Input: part model. Units: mm. Frame: model coordinates. Face numbers are marked on the shaded views. Coordinates: 2 decimals unless noted, no trailing zeros. Order: outer loops, then holes, each group sorted by start corner. A loop starts at its lowest first (then second) coordinate and runs counter-clockwise, first axis right, second up. Notation, with made-up numbers: M 58,-16 L 81,-16 A29 cw 81,9 Z; hole C -21,-34.5 d1. An arc over 180 degrees is marked long. Answer in a Markdown table with one row per item.
Autodesk Inventor part; units mm, degrees
ref_plane "YZ Plane" through (0, 0, 0) normal (1, 0, 0) x (0, 1, 0)
ref_plane "XZ Plane" through (0, 0, 0) normal (0, 1, 0) x (-1, 0, 0)
ref_plane "XY Plane" through (0, 0, 0) normal (0, 0, 1) x (1, 0, 0)
sketch "Sketch2" plane through (0, 0, 0) normal (1, 0, 0) x (0, 1, 0)
  circle A0 centre (0, 0) radius 10
  circle A1 centre (0, 0) radius 12.5
  dimension "d3" = 20
  dimension "d4" = 25
extrude "Extrusion1" add sketch "Sketch2" along normal blind 25
sketch "Sketch3" plane through (0, 0, 0) normal (-1, 0, 0) x (0, 0, 1)
  circle A0 centre (0, 0) radius 10
  arc A1 (10, 0) -> (-10, 0) centre (0, 0) ccw
  circle A2 centre (0, 0) radius 12.5
  arc A3 (12.5, 0) -> (-12.5, 0) centre (0, 0) ccw
  line L0 (-12.5, 0) -> (-10, 0)
  line L1 (10, 0) -> (12.5, 0)
revolve "Revolution1" add sketch "Sketch3" angle 180 about axis through (0, 0, 10) along (0, 0, 1) picked at (-11.4487, 1.7949) contours A0 L0 A2 L1
sketch "Sketch5" plane through (25, 0, 0) normal (1, 0, 0) x (0, 0, -1)
  circle A0 centre (-8, 8) radius 1
  point P0 (0, 0)
  dimension "d9" = 2
extrude "Extrusion2" add sketch "Sketch5" along normal blind 7
mirror "Mirror1" about plane through (0, 0, 0) normal (0, 0, 1) of "Extrusion2"
mirror "Mirror2" about plane through (0, 0, 0) normal (0, 1, 0) of "Extrusion2", "Mirror1"
properties part number "Plasmid Half 1"
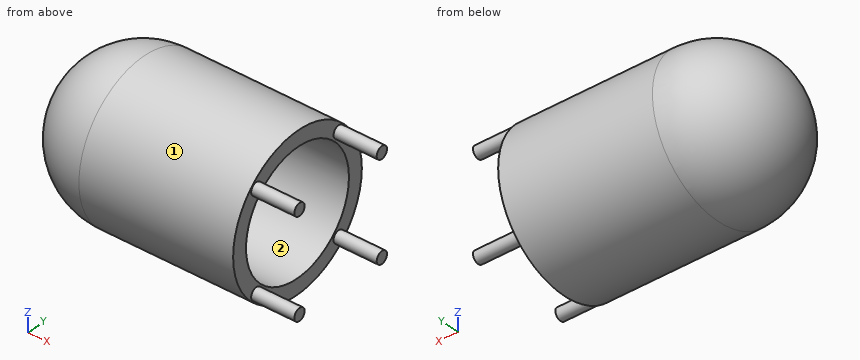
1) Contact query for flat-ended pins moving along their axis: pin 1 (4 mm diameter, centred on x = 4, y = 7, fed in from +Z); pin 2 (8 mm diameter, centred on y = -5, z = -2, fed in from -X); pin 3 (4 mm diameter, centred on x = 10, y = 9.5, fed in from -Z). Output: stop coordinate, or through.
Resolved:
| item | result |
|---|---|
| pin 1 | stops at z = 11.46 |
| pin 2 | stops at x = -12.42 |
| pin 3 | stops at z = -10 |
2) Cut plane A-A, the plane z = 0. Output: boundary loops of the cut face in (x, y).
Resolved:
| item | result |
|---|---|
| outline | M 0,-12.5 L 25,-12.5 L 25,-10 L 0,-10 A10 cw 0,10 L 25,10 L 25,12.5 L 0,12.5 A12.5 ccw Z |
3) Cut plane C-C, the plane x = 29.5. Output: boundary loops of the cut face in (y, z).
Resolved:
| item | result |
|---|---|
| outline | C -8,-8 d2; C -8,8 d2; C 8,-8 d2; C 8,8 d2 |
4) Mould query, pull axis Z, two halves, no side actions, for the marked faces 1 and 2. Classes: +Z half, -Z half, draft (parallel to the pull), parting line (faces both ways), or undercut.
Resolved:
| item | result |
|---|---|
| face 1 | parting line |
| face 2 | undercut |
5) Cut plane D-D, the plane y = -8. Output: boundary loops of the cut face in (x, z), and give its area (3 significant figures).
Resolved:
| item | result |
|---|---|
| outline | M 0,-9.6 L 25,-9.6 L 25,-9 L 32,-9 L 32,-7 L 25,-7 L 25,-6 L 0,-6 A6 cw 0,6 L 25,6 L 25,7 L 32,7 L 32,9 L 25,9 L 25,9.6 L 0,9.6 A9.6 ccw Z |
| area | 297 mm2 |
6) Material intervals for probe 1 along Z at (x, y) = (18.25, 0); probe 2 along Z at (x, y) = (-5, -1.75), sorted ascending.
Resolved:
| item | result |
|---|---|
| probe 1 | z = -12.5 to -10, 10 to 12.5 |
| probe 2 | z = -11.32 to -8.48, 8.48 to 11.32 |
